Part model, mm, in its own coordinate system. Round coordinates to 2 decimals unless told otherwise and drop trailing zeros. Loops run counter-clockwise (first coordinate to the right, second up) from the corner with the lowest first, then second, coordinate; pieces in that order, holes last.
1) Band-saw the part on B-B, the plane z = -5. Write the cut outline in (x, y), then the cut area to 3 significant figures.
2) Drop flat-ended pins along their axis: P1, Ø2.5, axis at x = -12, z = -5, coming from the -Y side; P2, Ø1.5, axis at x = -5.5, y = 2.5, coming from the -Z side; P3, Ø1.2, axis at x = 12, z = -5, coming from the +Y side. Give the stop position or say it passes through.
3) Band-saw the part on C-C, the plane y = 2.3. Write the cut outline in (x, z), then the cut area to 3 significant figures.
4) Band-saw the part on A-A, the plane x = 12. Write the cut outline in (y, z).
5) Band-saw the part on D-D, the plane z = -15. Write the cut outline in (x, y).
6) Probe line 1 (X direction, y = 0.8, z = -5); line 2 (X direction, y = 1.85, z = -24); line 3 (Z direction, x = 12, y = 1.9). List the from-to ranges inside material, lowest first.
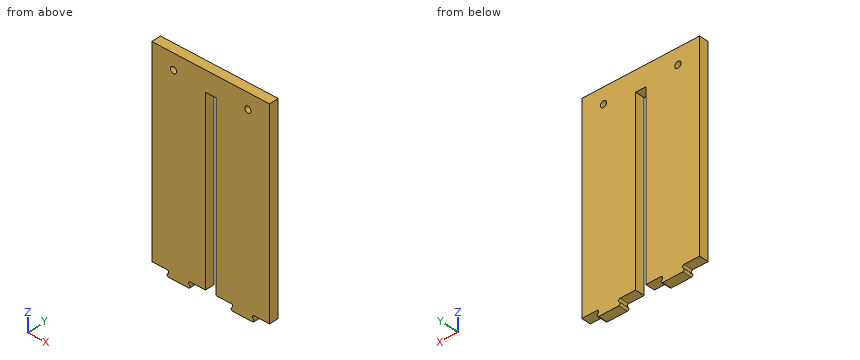
from build123d import *

# Parameters (mm, degrees)
SKETCH1_W           = 38
SKETCH1_H           = 72.5
BOSS_EXTRUDE1_DEPTH = 3.05
SKETCH4_W           = 1.65
SKETCH4_H           = 1
SKETCH4_H_2         = 61.8
CUT_EXTRUDE1_DEPTH  = 76.010349286
SKETCH7_R           = 1
CUT_EXTRUDE4_DEPTH  = 76.010349286
SKETCH8_W           = 38
SKETCH8_H           = 8.3
CUT_EXTRUDE5_DEPTH  = 76.010349286
BOSS_EXTRUDE3_DEPTH = 3.05
FILLET2_R           = 0.5


with BuildPart() as part:
    # Sketch1 → Boss-Extrude1 (new body)
    with BuildSketch(Plane(origin=(0, 0, 0), x_dir=(1, 0, 0), z_dir=(0, 1, 0))):
        with Locations((0, 36.25)):
            Rectangle(SKETCH1_W, SKETCH1_H)
    extrude(amount=BOSS_EXTRUDE1_DEPTH)

    # Sketch4 → Cut-Extrude1 (cut, through all)
    with BuildSketch(Plane(origin=(0, 3.05, 0), x_dir=(1, 0, 0), z_dir=(0, 1, 0))):
        with Locations((-0.825, 70)):
            Rectangle(SKETCH4_W, SKETCH4_H)
        with Locations((-0.825, 37.4)):
            Rectangle(SKETCH4_W, SKETCH4_H_2)
        with Locations((0.825, 37.4)):
            Rectangle(SKETCH4_W, SKETCH4_H_2)
        with Locations((0.825, 70)):
            Rectangle(SKETCH4_W, SKETCH4_H)
    extrude(amount=-CUT_EXTRUDE1_DEPTH, mode=Mode.SUBTRACT)

    # Sketch7 → Cut-Extrude4 (cut, through all)
    with BuildSketch(Plane(origin=(0, 3.05, 0), x_dir=(1, 0, 0), z_dir=(0, 1, 0))):
        with Locations(Location((-12, 5, 0), (0, 0, 270))):
            Circle(SKETCH7_R)
        with Locations(Location((12, 5, 0), (0, 0, 90))):
            Circle(SKETCH7_R)
    extrude(amount=-CUT_EXTRUDE4_DEPTH, mode=Mode.SUBTRACT)

    # Sketch8 → Cut-Extrude5 (cut, through all)
    with BuildSketch(Plane(origin=(0, 3.05, 0), x_dir=(1, 0, 0), z_dir=(0, 1, 0))):
        with Locations((0, 68.35)):
            Rectangle(SKETCH8_W, SKETCH8_H)
    extrude(amount=-CUT_EXTRUDE5_DEPTH, mode=Mode.SUBTRACT)

    # Sketch9 → Boss-Extrude3 (add)
    with BuildSketch(Plane(origin=(0, 3.05, 0), x_dir=(1, 0, 0), z_dir=(0, 1, 0))):
        Polygon((-14.575, 66.2), (-13, 64.2), (-7.65, 64.2), (-6.075, 66.2), align=None)
        Polygon((6.075, 66.2), (7.65, 64.2), (13, 64.2), (14.575, 66.2), align=None)
    extrude(amount=-BOSS_EXTRUDE3_DEPTH)

    # Fillet2
    fillet2_edges = [part.edges().sort_by_distance(p)[0] for p in [
        (-6.075, 1.525, -66.2),
        (-7.65, 1.525, -64.2),
        (-13, 1.525, -64.2),
        (-14.575, 1.525, -66.2),
        (14.575, 1.525, -66.2),
        (13, 1.525, -64.2),
        (7.65, 1.525, -64.2),
        (6.075, 1.525, -66.2),
    ]]
    fillet(fillet2_edges, radius=FILLET2_R)


solid = part.part
Reported:
1. outline: (-19, 0) - (-13, 0) - (-13, 3.05) - (-19, 3.05) - close; (-11, 0) - (11, 0) - (11, 3.05) - (-11, 3.05) - close; (13, 0) - (19, 0) - (19, 3.05) - (13, 3.05) - close
1. area: 104 mm2
2. P1: stops at y = 0
2. P2: stops at z = -64.2
2. P3: passes through
3. outline: (-19, -64.2) - (-14.03, -64.2) arc R0.5 cw to (-13.64, -65.01) - (-13.94, -65.39) arc R0.5 ccw to (-13.54, -66.2) - (-7.11, -66.2) arc R0.5 ccw to (-6.71, -65.39) - (-7.01, -65.01) arc R0.5 cw to (-6.62, -64.2) - (-1.65, -64.2) - (-1.65, -6.5) - (1.65, -6.5) - (1.65, -64.2) - (6.62, -64.2) arc R0.5 cw to (7.01, -65.01) - (6.71, -65.39) arc R0.5 ccw to (7.11, -66.2) - (13.54, -66.2) arc R0.5 ccw to (13.94, -65.39) - (13.64, -65.01) arc R0.5 cw to (14.03, -64.2) - (19, -64.2) - (19, 0) - (-19, 0) - close; hole circle Ø2 at (-12, -5); hole circle Ø2 at (12, -5)
3. area: 2,270 mm2
4. outline: (0, -66.2) - (3.05, -66.2) - (3.05, -6) - (0, -6) - close; (0, -4) - (3.05, -4) - (3.05, 0) - (0, 0) - close
5. outline: (-19, 0) - (-1.65, 0) - (-1.65, 3.05) - (-19, 3.05) - close; (1.65, 0) - (19, 0) - (19, 3.05) - (1.65, 3.05) - close
6. line 1: x = -19 to -13, -11 to 11, 13 to 19
6. line 2: x = -19 to -1.65, 1.65 to 19
6. line 3: z = -66.2 to -6, -4 to 0
